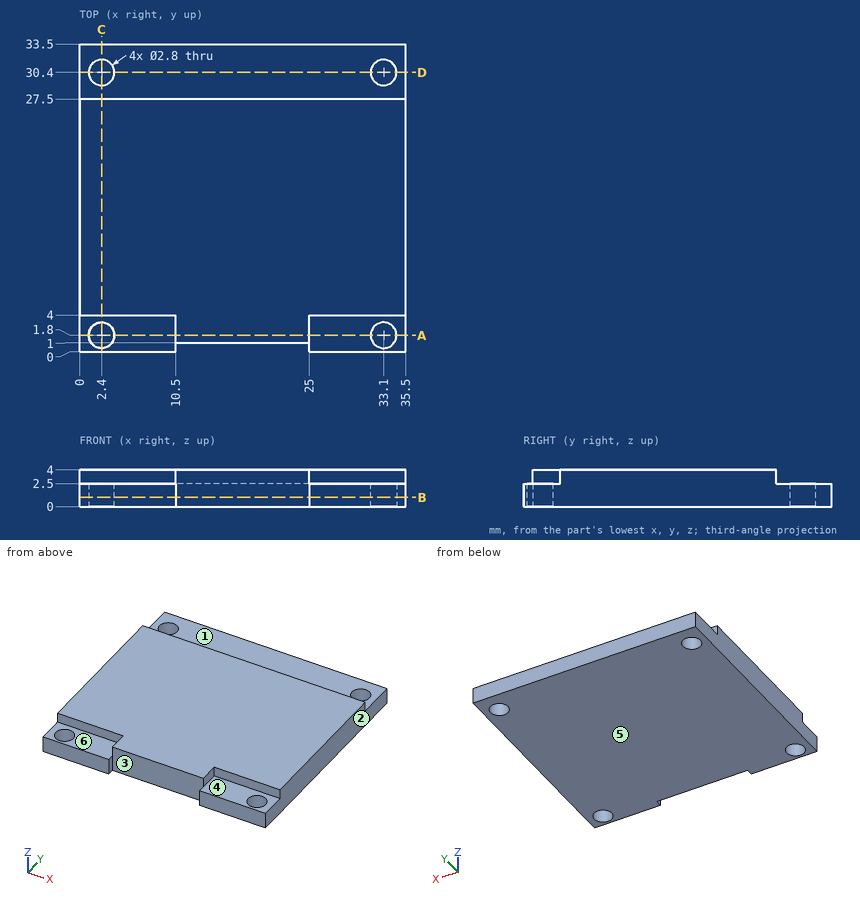
Print and shaded views of the part. All mm, measured from the part's lowest x, y and z. A direction names the side the tool comes from. Coordinates: 2 decimals unless noted, no trailing zeros. Loops run counter-clockwise (first coordinate to the right, second up) from the corner with the lowest first, then second, coordinate; pieces in that order, holes last. Notation, with made-up numbers: (-32.75, 50) -> (-27.75, 50) arc R11 ccw to (-27.75, 62) -> close; hole circle Ø10 at (38.25, 28). An arc over 180 degrees is marked (long way). Use one line per item in the form item = value. Start each with the question number.
(1) Pull direction X, two halves, no side cores. Call the marked faces 1, 2 and 3: pulls with the +X half, pulls with the -X half, needs draft (parallel to the pull), parting line crosses it, or undercut.
(2) Cut at B-B on z = 1. Give the cut face in (x, y), and give its area (3 significant figures).
(3) Cut at D-D on y = 30.4. Give the cut face in (x, z).
(4) Cut at C-C on x = 2.4. Give the cut face in (y, z), and give its area (3 significant figures).
(5) Tool access for the marked faces 4, 5 and 6: list every direction of +Z, -Z, +X, -X, +Y, -Y with a clear straight run to the whole face (end or side of a thin tool).
(6) Probe probe 1 along Y at (x, z) = (2.4, 0.9); probe 2 along Y at (x, z) = (24, 0.2); probe 3 along Y at (x, z) = (18, 3.25). List the from-to ranges inside material, lowest first. Write a range as from..to.
(7) Cut at A-A on y = 1.8. Give the cut face in (x, z), and give its area (3 significant figures).
(8) Flat gauge pins, fed straight in: pin 1 (1.1 mm diameter, centred on y = 0.5, z = 1, fed in from -X); pin 2 (1.6 mm diameter, centred on x = 9.5, z = 3.5, fed in from +Y); pin 3 (1 mm diameter, centred on x = 17.5, z = 1, fed in from -Y); pin 4 (3 mm diameter, centred on x = 28, y = 2, fed in from +Z). Where does each tip first touch, or does it go through?
Values:
q1.face_1 = needs draft
q1.face_2 = pulls with the +X half
q1.face_3 = undercut
q2.outline = (0, 0) -> (10.5, 0) -> (10.5, 1) -> (25, 1) -> (25, 0) -> (35.5, 0) -> (35.5, 33.5) -> (0, 33.5) -> close; hole circle Ø2.8 at (2.4, 1.8); hole circle Ø2.8 at (2.4, 30.4); hole circle Ø2.8 at (33.1, 1.8); hole circle Ø2.8 at (33.1, 30.4)
q2.area = 1,150 mm2
q3.outline = (0, 0) -> (1, 0) -> (1, 2.5) -> (0, 2.5) -> close; (3.8, 0) -> (31.7, 0) -> (31.7, 2.5) -> (3.8, 2.5) -> close; (34.5, 0) -> (35.5, 0) -> (35.5, 2.5) -> (34.5, 2.5) -> close
q4.outline = (0, 0) -> (0.4, 0) -> (0.4, 2.5) -> (0, 2.5) -> close; (3.2, 0) -> (29, 0) -> (29, 2.5) -> (27.5, 2.5) -> (27.5, 4) -> (4, 4) -> (4, 2.5) -> (3.2, 2.5) -> close; (31.8, 0) -> (33.5, 0) -> (33.5, 2.5) -> (31.8, 2.5) -> close
q4.area = 105 mm2
q5.face_4 = +Z, +X, -Y
q5.face_5 = -Z, +X, -X, +Y, -Y
q5.face_6 = +Z, -X, -Y
q6.probe_1 = 0..0.4, 3.2..29, 31.8..33.5
q6.probe_2 = 1..33.5
q6.probe_3 = 1..27.5
q7.outline = (0, 0) -> (1, 0) -> (1, 2.5) -> (0, 2.5) -> close; (3.8, 0) -> (31.7, 0) -> (31.7, 2.5) -> (25, 2.5) -> (25, 4) -> (10.5, 4) -> (10.5, 2.5) -> (3.8, 2.5) -> close; (34.5, 0) -> (35.5, 0) -> (35.5, 2.5) -> (34.5, 2.5) -> close
q7.area = 96.5 mm2
q8.pin_1 = 0
q8.pin_2 = 27.5
q8.pin_3 = 1
q8.pin_4 = 2.5
